Print and shaded views of the part. All mm, measured from the part's lowest x, y and z. A direction names the side the tool comes from. Round coordinates to 2 decimals unless told otherwise and drop trailing zeros. Order: outer loops, then holes, each group sorted by start corner. A loop starts at its lowest first (then second) coordinate and runs counter-clockwise, first axis right, second up. Notation, with made-up numbers: M -5,-37.5 L 52,-37.5 A26 ccw 52,-11.5 Z; hole C 20.5,64 d8. An arc over 180 degrees is marked long. Write each question's results on one line, items separated by ' | '. Start each with the question number.
1. Probe L1, parallel to Z at x = 16, y = 5.5; L2, parallel to Z at x = 28, y = 16.5 (1 decimal); L3, parallel to X at y = 22, z = 18.75. List the from-to ranges inside material, lowest first. Write a range as [from, to].
2. Band-saw the part on B-B, the plane y = 38. List the corners of the cut face in (x, z) (1 decimal).
3. Band-saw the part on A-A, the plane x = 6. List the corners of the cut face in (y, z) (1 decimal).
4. Band-saw the part on D-D, the plane x = 27. List the corners of the cut face in (y, z) (1 decimal).
5. Two-plate mould, pull along X, no slides. Class the marked faces 4, 5 and 6: +X half, -X half, draft (parallel to the pull), parting line (faces both ways), or undercut.
6. Drop flat-ended pins along their axis: pin 1 Ø2 at (x, z) = (9.5, 16.5) entering from -Y; pin 2 Ø6 at (x, y) = (32, 10.5) entering from +Z; pin 3 Ø2 at (x, z) = (15.5, 12) entering from -Y (1 decimal); pin 4 Ø5 at (x, z) = (28, 24) entering from -Y (1 decimal). Give the stop position or say it passes through.
7. Which spindle directions (+Z, -Z, +X, -X, +Y, -Y) get a long thin tool onto all of the face, cutting with end or side? Do the marked faces 1, 2 and 3. Say none if no direction does.
8. Band-saw the part on C-C, the plane y = 19. List the corners of the cut face in (x, z) (1 decimal).
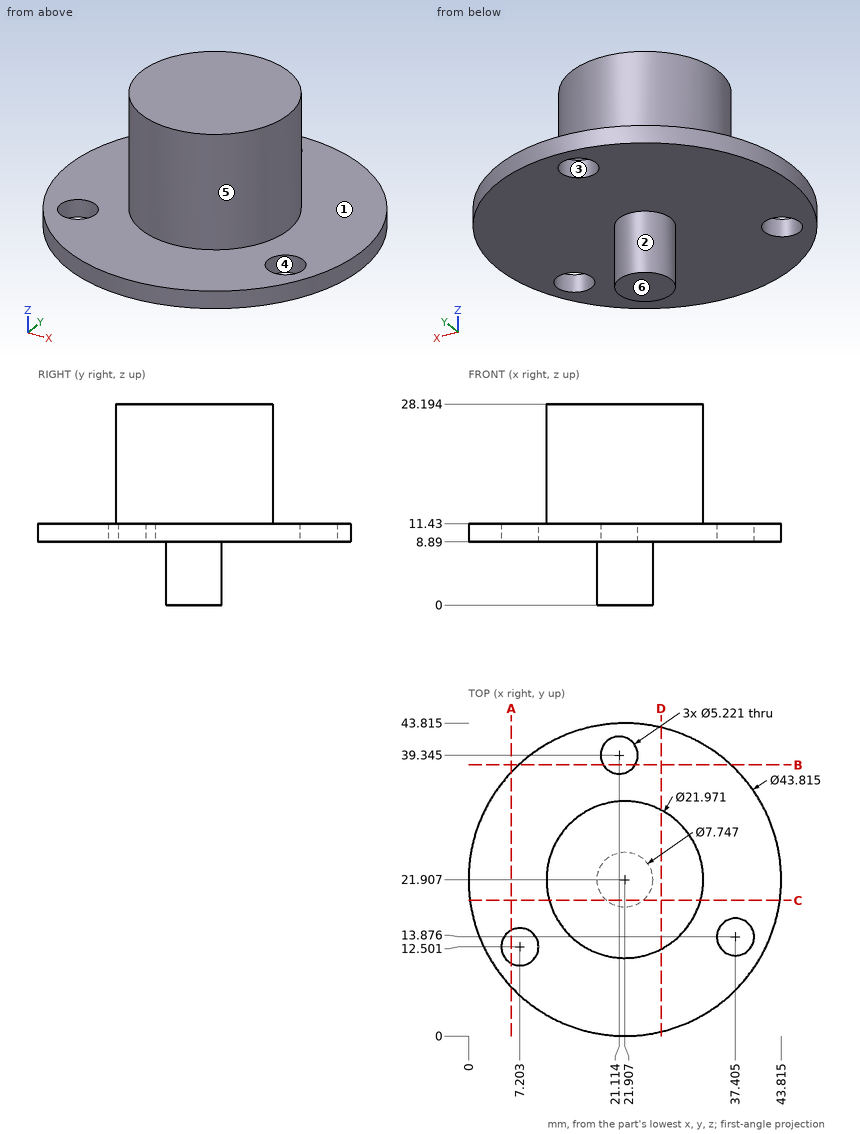
Solution:
1) L1: [8.89, 11.43] | L2: [8.9, 28.2] | L3: [10.92, 32.89]
2) outline: M 7,8.9 L 18.9,8.9 L 18.9,11.4 L 7,11.4 Z; M 23.4,8.9 L 36.8,8.9 L 36.8,11.4 L 23.4,11.4 Z
3) outline: M 6.8,8.9 L 10.2,8.9 L 10.2,11.4 L 6.8,11.4 Z; M 14.8,8.9 L 37,8.9 L 37,11.4 L 14.8,11.4 Z
4) outline: M 0.6,8.9 L 43.2,8.9 L 43.2,11.4 L 31.6,11.4 L 31.6,28.2 L 12.2,28.2 L 12.2,11.4 L 0.6,11.4 Z
5) face 4: undercut | face 5: parting line | face 6: draft
6) pin 1: through | pin 2: z = 11.43 | pin 3: y = 0.7 | pin 4: y = 11.5
7) face 1: +Z | face 2: -Z | face 3: +Z, -Z
8) outline: M 0.2,8.9 L 19.3,8.9 L 19.3,0 L 24.5,0 L 24.5,8.9 L 43.6,8.9 L 43.6,11.4 L 32.5,11.4 L 32.5,28.2 L 11.3,28.2 L 11.3,11.4 L 0.2,11.4 Z
